from build123d import *

# Parameters (mm, degrees)
CROQUIS1_R                     = 11
CROQUIS1_R_2                   = 9.5
SALIENTE_EXTRUIR1_DEPTH        = 4
SALIENTE_EXTRUIR1_DEPTH_BACK   = 4
CROQUIS1_R_3                   = 5.5
CROQUIS1_R_4                   = 4
SALIENTE_EXTRUIR1_2_DEPTH      = 4
SALIENTE_EXTRUIR1_2_DEPTH_BACK = 4
CROQUIS1_4_R                   = 9.5
CROQUIS1_4_R_2                 = 5.5
SALIENTE_EXTRUIR2_DEPTH        = 3.5
SALIENTE_EXTRUIR2_DEPTH_BACK   = 3.5


with BuildPart() as part:
    # Croquis1 → Saliente-Extruir1 (new body, two sides)
    with BuildSketch(Plane.XY) as saliente_extruir1_sk:
        Circle(CROQUIS1_R)
        Circle(CROQUIS1_R_2, mode=Mode.SUBTRACT)
    extrude(amount=SALIENTE_EXTRUIR1_DEPTH)
    extrude(saliente_extruir1_sk.sketch, amount=-SALIENTE_EXTRUIR1_DEPTH_BACK)



with BuildPart() as body_2:
    # Croquis1 → Saliente-Extruir1 2 (new body, two sides)
    with BuildSketch(Plane.XY) as saliente_extruir1_2_sk:
        Circle(CROQUIS1_R_3)
        Circle(CROQUIS1_R_4, mode=Mode.SUBTRACT)
    extrude(amount=SALIENTE_EXTRUIR1_2_DEPTH)
    extrude(saliente_extruir1_2_sk.sketch, amount=-SALIENTE_EXTRUIR1_2_DEPTH_BACK)


with BuildPart() as part_1:
    add(part.part)

    add(body_2.part)  # Saliente-Extruir2 merges body 2
    # Croquis1_4 → Saliente-Extruir2 (add, two sides)
    with BuildSketch(Plane.XY) as saliente_extruir2_sk:
        Circle(CROQUIS1_4_R)
        Circle(CROQUIS1_4_R_2, mode=Mode.SUBTRACT)
    extrude(amount=SALIENTE_EXTRUIR2_DEPTH)
    extrude(saliente_extruir2_sk.sketch, amount=-SALIENTE_EXTRUIR2_DEPTH_BACK)


solid = part_1.part
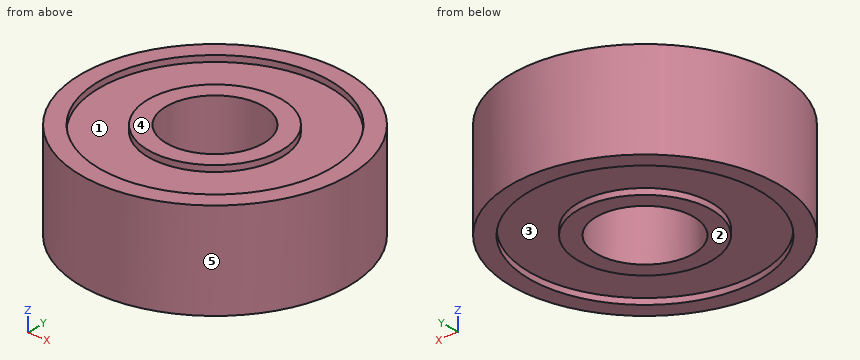
The listing builds one solid part. Answer for the finished solid, in the listing's coordinates (mm). Face numbers are marked on the shaded views. A direction names the side the tool comes from. Give positions to 0.01 mm unless a question says otherwise; leave off trailing zeros. Loops run counter-clockwise (first coordinate to the right, second up) from the corner with the lowest first, then second, coordinate; pieces in that order, holes last. Notation, with made-up numbers: (26, -38.5) - (85, -38.5) arc R5 cw to (85, -31.5) - close; hole circle Ø6 at (1.5, 80.5). An arc over 180 degrees is marked (long way). Use one line per item in the form item = value.
1. The mould has two halves that part along X. Classify the marked faces 3, 4 and 5: pulls with the +X half, pulls with the -X half, needs draft (parallel to the pull), parting line crosses it, or undercut.
Calculated:
face_3 = undercut
face_4 = needs draft
face_5 = parting line crosses it
2. Which of the six approach directions +Z, -Z, +X, -X, +Y, -Y give full straight-line access (tool end or side, diameter ignored) to the marked faces 1 and 2?
Calculated:
face_1 = +Z
face_2 = -Z, +X, -X, +Y, -Y
3. Given pin 1 Ø2 at (x, z) = (-1.5, 1) entering from +Y; pin 2 Ø1 at (x, y) = (-2.5, 8) entering from +Z; pin 3 Ø1 at (x, z) = (-2, -2) entering from +Y, each flat-ended and moving along its own axis, determine where each tip first touches the part or whether it passes through.
Calculated:
pin_1 = 10.99
pin_2 = 3.5
pin_3 = 10.9
4. Section A-A on y = 0 is taken. Give the vertices of the cut face in (x, z).
Calculated:
outline = (-11, -4) - (-9.5, -4) - (-9.5, -3.5) - (-5.5, -3.5) - (-5.5, -4) - (-4, -4) - (-4, 4) - (-5.5, 4) - (-5.5, 3.5) - (-9.5, 3.5) - (-9.5, 4) - (-11, 4) - close; (4, -4) - (5.5, -4) - (5.5, -3.5) - (9.5, -3.5) - (9.5, -4) - (11, -4) - (11, 4) - (9.5, 4) - (9.5, 3.5) - (5.5, 3.5) - (5.5, 4) - (4, 4) - close
5. Section D-D on y = -9 is taken. Give the vertices of the cut face in (x, z).
Calculated:
outline = (-6.32, -4) - (-3.04, -4) - (-3.04, -3.5) - (3.04, -3.5) - (3.04, -4) - (6.32, -4) - (6.32, 4) - (3.04, 4) - (3.04, 3.5) - (-3.04, 3.5) - (-3.04, 4) - (-6.32, 4) - close
6. Section C-C on z = 1.5 is taken. Give the vertices of the cut face in (x, y), then the cut area to 3 significant figures.
Calculated:
outline = circle Ø22 at (0, 0); hole circle Ø8 at (0, 0)
area = 330 mm^2
7. Find the intervals of material crossed by line 1 along Y through (x, z) = (0, -3.75); line 2 along Y through (x, z) = (0, -0.25); line 3 along Z through (x, y) = (-3.25, 8.25), in increasing order. Write a range as [from, to].
Calculated:
line_1 = [-11, -9.5], [-5.5, -4], [4, 5.5], [9.5, 11]
line_2 = [-11, -4], [4, 11]
line_3 = [-3.5, 3.5]
